Verification items for the finished model (mm, model axes). Give positions to 0.01 mm unless a question says otherwise; leave off trailing zeros. Loops run counter-clockwise (first coordinate to the right, second up) from the corner with the lowest first, then second, coordinate; pieces in that order, holes last. Notation, with made-up numbers: (18.25, 48) - (43.25, 48) arc R27 ccw to (43.25, 68) - close; hole circle Ø2 at (25.5, 47). An arc over 180 degrees is marked (long way). Put each result on its own line as item: value. Start each with the question number.
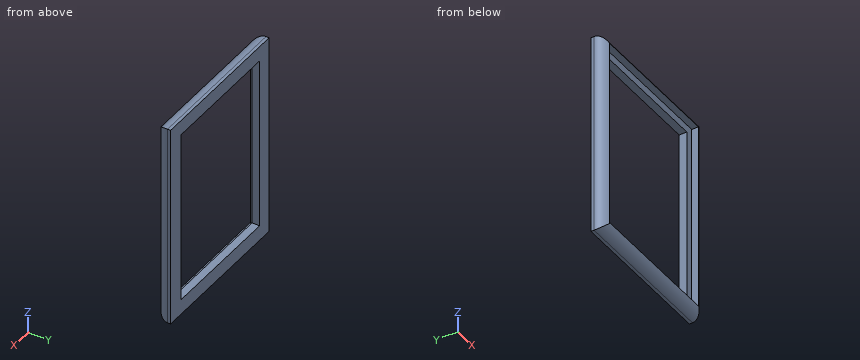
```python
from build123d import *

# Parameters (mm, degrees)
F0_W        = 200
F0_H        = 270
F1_DEPTH    = 20
F2_W        = 180
F2_H        = 250
F3_DEPTH    = 10
F4_W        = 160
F4_H        = 230
F5_DEPTH    = 25
F6_T1_DEPTH = 350
F6_T3_DEPTH = 280


# Not quite as in the source:
# - a fillet or chamfer that OpenCascade refuses, or shapes differently, is made with other operations: its cross-section is extruded or revolved along the edge and cut away or added


with BuildPart() as f1:
    # F0 (on Front) → F1 (new body)
    with BuildSketch(Plane.XZ):
        with Locations((-21.7714021464, 1.2882190198)):
            Rectangle(F0_W, F0_H)
    extrude(amount=F1_DEPTH)

    # F2 (on face) → F3 (cut)
    with BuildSketch(Plane.XZ.offset(20)):
        with Locations((-22.5493634492, 1.4232655292)):
            Rectangle(F2_W, F2_H)
    extrude(amount=-F3_DEPTH, mode=Mode.SUBTRACT)

    # F4 (on face) → F5 (cut)
    with BuildSketch(Plane.XZ.offset(10)):
        with Locations((-22.5493634492, 1.4232655292)):
            Rectangle(F4_W, F4_H)
    extrude(amount=-F5_DEPTH, mode=Mode.SUBTRACT)

    # F6: fillet of radius 16 on 4 edges, made by hand

    # F6_s2 → F6_t1 (cut)
    with BuildSketch(Plane.XY.offset(-173.7117809802)):
        with BuildLine():
            ThreePointArc((-121.7714021464, -4), (-117.0851106454, -15.313708499), (-105.7714021464, -20))
            Line((-105.7714021464, -20), (-121.7714021464, -20))
            Line((-121.7714021464, -20), (-121.7714021464, -4))
        make_face()
        with BuildLine():
            ThreePointArc((62.2285978536, -20), (73.5423063526, -15.313708499), (78.2285978536, -4))
            Line((78.2285978536, -4), (78.2285978536, -20))
            Line((78.2285978536, -20), (62.2285978536, -20))
        make_face()
    extrude(amount=F6_T1_DEPTH, mode=Mode.SUBTRACT)

    # F6_s4 → F6_t3 (cut)
    with BuildSketch(Plane.YZ.offset(-161.7714021464)):
        with BuildLine():
            ThreePointArc((-4, 136.2882190198), (-15.313708499, 131.6019275188), (-20, 120.2882190198))
            Line((-20, 120.2882190198), (-20, 136.2882190198))
            Line((-20, 136.2882190198), (-4, 136.2882190198))
        make_face()
        with BuildLine():
            ThreePointArc((-4, -133.7117809802), (-15.313708499, -129.0254894792), (-20, -117.7117809802))
            Line((-20, -117.7117809802), (-20, -133.7117809802))
            Line((-20, -133.7117809802), (-4, -133.7117809802))
        make_face()
    extrude(amount=F6_T3_DEPTH, mode=Mode.SUBTRACT)


solid = f1.part
```
1) Section check B-B, the plane z = -8. Enter the section's corners in (x, y), plus the area to 3 significant figures.
2) Depth check by flat-ended pin: P1, Ø10, axis at y = -15, z = 33, coming from the -X side; P2, Ø5, axis at y = -5.5, z = -5, coming from the -X side; P3, Ø4, axis at y = -14, z = -51.5, coming from the +X side (3 decimals); P4, Ø5, axis at y = -10.5, z = 20.5, coming from the -X side. Enter the tip coordinate at first touch or a pass-through.
3) Scan lines: line 1 along X through (y, z) = (-5, -58.5); line 2 along X through (y, z) = (-2.75, 62); line 3 along Z through (x, y) = (-39, -10.75). Record each from-to range of solid material in increasing order. Write a range as from..to.
4) Section check A-A, the plane x = -23. Enter the section's corners in (y, z).
5) Section check C-C, the plane x = 63. Enter the section's corners in (y, z), plus the area to 3 significant figures.
6) Section check D-D, the plane y = -13. Enter the section's corners in (x, z), plus the area to 3 significant figures.
Results are:
1. outline: (-121.77, -4) arc R16 ccw to (-112.55, -18.49) - (-112.55, -10) - (-102.55, -10) - (-102.55, 0) - (-121.77, 0) - close; (57.45, -10) - (67.45, -10) - (67.45, -19.12) arc R16 ccw to (78.23, -4) - (78.23, 0) - (57.45, 0) - close
1. area: 495 mm2
2. P1: stops at x = -120.6
2. P2: stops at x = -121.77
2. P3: stops at x = 76.085
2. P4: stops at x = -121.26
3. line 1: x = -121.74..-102.55, 57.45..78.2
3. line 2: x = -121.77..-102.55, 57.45..78.23
3. line 3: z = -132.22..-123.58, 126.42..134.79
4. outline: (-18.89, -123.58) arc R16 ccw to (-4, -133.71) - (0, -133.71) - (0, -113.58) - (-10, -113.58) - (-10, -123.58) - close; (-18.78, 126.42) - (-10, 126.42) - (-10, 116.42) - (0, 116.42) - (0, 136.29) - (-4, 136.29) arc R16 ccw to start
5. outline: (-18.89, -123.58) arc R16 ccw to (-4, -133.71) - (0, -133.71) - (0, 136.29) - (-4, 136.29) arc R16 ccw to (-18.78, 126.42) - (-10, 126.42) - (-10, -123.58) - close
5. area: 2,790 mm2
6. outline: (-119, -130.94) - (75.46, -130.94) - (75.46, 133.52) - (-119, 133.52) - close; hole (-112.55, -123.58) - (67.45, -123.58) - (67.45, 126.42) - (-112.55, 126.42) - close
6. area: 6,430 mm2
